Verification items for this drawing (mm, ordinates from the low corner). A direction names the side the tool comes from. Give positions to 0.01 mm unless a question says otherwise; leave off trailing zeros. Loops run counter-clockwise (first coordinate to the right, second up) from the corner with the lowest first, then second, coordinate; pieces in that order, holes last. Notation, with made-up numbers: (-39, 66.5) -> (-8, 66.5) arc R25 ccw to (-8, 89.5) -> close; hole circle Ø6 at (71.25, -29). An arc over 180 degrees is marked (long way). Answer in a Markdown table with one row per item. Add a question column.
Q1. Section check C-C on x = 54.5. Enter the section's corners in (y, z), and give its area (3 significant figures).
Q2. Gauge pin test, flat ends, axial feed: P1, Ø3, axis at x = 99, y = 4.5, coming from the -Z side (1 decimal); P2, Ø3, axis at y = 3, z = 37, coming from the +X side (3 decimals). Record the tip position at first contact, or that the pin passes through.
Q3. Section check A-A on y = 3.75. Enter the section's corners in (x, z).
Q4. Material ranges on probe 1 along X at (y, z) = (1, 5); probe 2 along Z at (x, y) = (61.5, 0.3); probe 3 along Y at (x, z) = (99.5, 59.5), recorded low to high.
Q5. Section check D-D on z = 78.5. Enter the section's corners in (x, y) (1 decimal).
Q6. Section check B-B on z = 103. Enter the section's corners in (x, y).
Q7. Set-up check for the marked faces 1 and 2: record each of +Z, -Z, +X, -X, +Y, -Y from which the full face is reachable in a straight line by a thin tool's end or side.
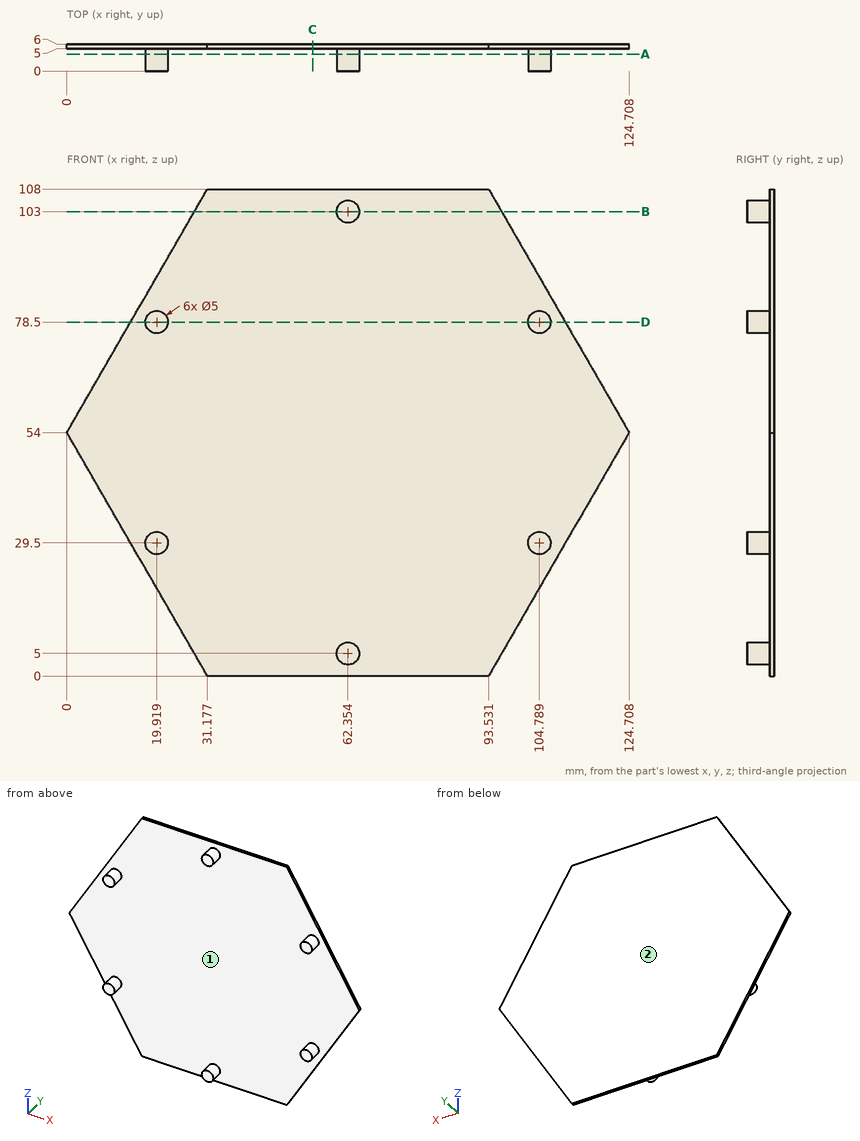
Taken from the geometry:
| question | item | result |
|---|---|---|
| 1 | outline | (5, 0) -> (6, 0) -> (6, 108) -> (5, 108) -> close |
| 1 | area | 108 mm² |
| 2 | P1 | stops at z = 7 |
| 2 | P2 | passes through |
| 3 | outline | circle Ø5 at (19.92, 29.5); circle Ø5 at (19.92, 78.5); circle Ø5 at (62.35, 5); circle Ø5 at (62.35, 103); circle Ø5 at (104.79, 29.5); circle Ø5 at (104.79, 78.5) |
| 4 | probe 1 | x = 59.85 to 64.85 |
| 4 | probe 2 | z = 2.65 to 7.35, 100.65 to 105.35 |
| 4 | probe 3 | y = 5 to 6 |
| 5 | outline | (14.1, 5) -> (17.4, 5) -> (17.4, 0) -> (22.4, 0) -> (22.4, 5) -> (102.3, 5) -> (102.3, 0) -> (107.3, 0) -> (107.3, 5) -> (110.6, 5) -> (110.6, 6) -> (14.1, 6) -> close |
| 6 | outline | (28.29, 5) -> (59.85, 5) -> (59.85, 0) -> (64.85, 0) -> (64.85, 5) -> (96.42, 5) -> (96.42, 6) -> (28.29, 6) -> close |
| 7 | face 1 | -Y |
| 7 | face 2 | +Z, -Z, +X, -X, +Y |
